Can you work these out from the model? Positions are in its coordinate system, mm. A direction names the side the tool comes from. Give positions to 0.01 mm unless a question says otherwise; leave off trailing zeros. Loops run counter-clockwise (first coordinate to the right, second up) from the corner with the lowest first, then second, coordinate; pieces in that order, holes last. Notation, with made-up numbers: (-12.5, 4.5) - (-2.5, 4.5) arc R19 cw to (-2.5, 31.5) - close; hole circle Ø2 at (32.25, 28). An arc over 180 degrees is marked (long way). Answer as a JSON object with one key per item and string values. Group by question number.
Item 1: Which directions (+Z, -Z, +X, -X, +Y, -Y) give clear straight access to the entire face, cutting with the end or side of a thin tool? Please do faces 1 (the flat face through (24.124, -8, 3)), 2 (the flat face through (13, 25.341, 3)), 3 (the flat face through (91.377, 57, 3)).
Item 2: Thinking about a two-plate mould opening in Y: for faces 4 (the flat face through (90.772, -8, 3)), 5 (the flat face through (48.223, 98.615, 2.958)), 6 (the flat face through (32.043, 67, 3)), which applies, pulls with the +Y half, pulls with the -Y half, needs draft (parallel to the pull), parting line crosses it, or undercut?
Item 3: Suppose I cut it at C-C on z = 2.9. Count the separate pieces of the cut face and the enclosed holes in it, and give its area (3 significant figures).
Item 4: Suppose I cut it at D-D on y = 30. Write out the boundary of the cut face in (x, z).
Item 5: Please list where these lines run through material, in increasing order: L1, parallel to Y at x = 10, z = 3.25; L2, parallel to Y at x = 34.5, z = 3.95; L3, parallel to Y at x = 56.5, z = 5.1.
Item 6: Will these pins go through, and if not, where does the flat tip stop? pin 1 (1.8 mm diameter, centred on y = -7.5, z = 3.5, fed in from +X); pin 2 (2.5 mm diameter, centred on x = 10, z = 4.5, fed in from -Y); pin 3 (1.5 mm diameter, centred on x = 82, z = 2.5, fed in from +Y).
Item 7: Suppose I cut it at B-B on y = 67.5. Write out the boundary of the cut face in (x, z).
Item 8: Suppose I cut it at A-A on x = 14.5. Write out the boundary of the cut face in (y, z).
from build123d import *

# Parameters (mm, degrees)
SKETCH1_W           = 12.2
SKETCH1_H           = 23
BOSS_EXTRUDE1_DEPTH = 6


with BuildPart() as part:
    # Sketch1 → Boss-Extrude1 (new body)
    with BuildSketch(Plane.XY):
        with BuildLine():
            Line((21.077436259, 96.487236066), (24.514288944, 100.118770675))
            ThreePointArc((24.514288944, 100.118770675), (26.133905044, 101.250028723), (28.068821983, 101.648773655))
            Line((28.068821983, 101.648773655), (30.683177697, 101.648773655))
            Line((30.683177697, 101.648773655), (30.683177697, 96.648773655))
            Line((30.683177697, 96.648773655), (33.683177697, 96.648773655))
            Line((33.683177697, 96.648773655), (33.683177697, 101.648773655))
            Line((33.683177697, 101.648773655), (43.068821983, 101.648773655))
            ThreePointArc((43.068821983, 101.648773655), (44.879241743, 101.301597143), (46.432801053, 100.309324643))
            Line((46.432801053, 100.309324643), (50.064335662, 96.872471958))
            ThreePointArc((50.064335662, 96.872471958), (51.617894972, 95.880199458), (53.428314733, 95.533022946))
            Line((53.428314733, 95.533022946), (55.683177697, 95.533022946))
            Line((55.683177697, 95.533022946), (55.683177697, 90.533022946))
            Line((55.683177697, 90.533022946), (58.683177697, 90.533022946))
            Line((58.683177697, 90.533022946), (58.683177697, 95.533022946))
            Line((58.683177697, 95.533022946), (61.489325132, 95.533022946))
            ThreePointArc((61.489325132, 95.533022946), (62.461477954, 95.280855573), (63.188485552, 94.587941837))
            Line((63.188485552, 94.587941837), (66.784051646, 88.796554795))
            ThreePointArc((66.784051646, 88.796554795), (67.511059245, 88.10364106), (68.483212066, 87.851473686))
            Line((68.483212066, 87.851473686), (80.727367549, 87.851473686))
            Line((80.727367549, 87.851473686), (80.727367549, 82.851473686))
            Line((80.727367549, 82.851473686), (83.727367549, 82.851473686))
            Line((83.727367549, 82.851473686), (83.727367549, 87.851473686))
            Line((83.727367549, 87.851473686), (93.887367549, 87.851473686))
            ThreePointArc((93.887367549, 87.851473686), (97.660193959, 86.132598628), (98.839013483, 82.157786039))
            Line((98.839013483, 82.157786039), (90.771737035, 1.27912723))
            Line((90.771737035, 1.27912723), (90.771737035, -16.699114739))
            Line((90.771737035, -16.699114739), (80.611737035, -16.699114739))
            Line((80.611737035, -16.699114739), (80.611737035, 1.27912723))
            Line((80.611737035, 1.27912723), (75.531737035, 1.27912723))
            Line((75.531737035, 1.27912723), (75.531737035, -16.699114739))
            Line((75.531737035, -16.699114739), (67.911737035, -16.699114739))
            Line((67.911737035, -16.699114739), (67.911737035, 1.27912723))
            Line((67.911737035, 1.27912723), (62.831737035, 1.27912723))
            Line((62.831737035, 1.27912723), (62.831737035, -16.699114739))
            Line((62.831737035, -16.699114739), (24.124020717, -16.699114739))
            Line((24.124020717, -16.699114739), (24.124020717, 1.27912723))
            Line((24.124020717, 1.27912723), (19.044020717, 1.27912723))
            Line((19.044020717, 1.27912723), (19.044020717, -16.699114739))
            Line((19.044020717, -16.699114739), (11.424020717, -16.699114739))
            Line((11.424020717, -16.699114739), (11.424020717, 1.27912723))
            Line((11.424020717, 1.27912723), (6.344020717, 1.27912723))
            Line((6.344020717, 1.27912723), (6.344020717, -16.699114739))
            Line((6.344020717, -16.699114739), (-3.815979283, -16.699114739))
            Line((-3.815979283, -16.699114739), (-3.815979283, 1.27912723))
            Line((-3.815979283, 1.27912723), (-3.815979283, 10.864597722))
            Line((-3.815979283, 10.864597722), (8.569519397, 16.399351506))
            Line((8.569519397, 16.399351506), (8.569519397, 20.261157087))
            Line((8.569519397, 20.261157087), (17.062273891, 20.261157087))
            Line((17.062273891, 20.261157087), (17.062273891, 25.341157087))
            Line((17.062273891, 25.341157087), (8.569519397, 25.341157087))
            Line((8.569519397, 25.341157087), (8.569519397, 32.909351506))
            Line((8.569519397, 32.909351506), (17.062273891, 32.909351506))
            Line((17.062273891, 32.909351506), (17.062273891, 37.989351506))
            Line((17.062273891, 37.989351506), (8.569519397, 37.989351506))
            Line((8.569519397, 37.989351506), (8.569519397, 41.799351506))
            Line((8.569519397, 41.799351506), (-3.815979283, 49.840454802))
            Line((-3.815979283, 49.840454802), (-7.075944103, 93.020454802))
            ThreePointArc((-7.075944103, 93.020454802), (-5.26079125, 95.528652506), (-2.316822303, 96.487236066))
            Line((-2.316822303, 96.487236066), (5.683177697, 96.487236066))
            Line((5.683177697, 96.487236066), (5.683177697, 91.487236066))
            Line((5.683177697, 91.487236066), (8.683177697, 91.487236066))
            Line((8.683177697, 91.487236066), (8.683177697, 96.487236066))
            Line((8.683177697, 96.487236066), (21.077436259, 96.487236066))
        make_face()
        with Locations((85.276683747, 57.465671264)):
            Rectangle(SKETCH1_W, SKETCH1_H, mode=Mode.SUBTRACT)
        with Locations((62.066293543, 63.009787098)):
            Rectangle(SKETCH1_W, SKETCH1_H, mode=Mode.SUBTRACT)
        with Locations((38.142588603, 67.50121976)):
            Rectangle(SKETCH1_W, SKETCH1_H, mode=Mode.SUBTRACT)
        with Locations((12.98270306, 64.099542403)):
            Rectangle(SKETCH1_W, SKETCH1_H, mode=Mode.SUBTRACT)
    extrude(amount=BOSS_EXTRUDE1_DEPTH)


solid = part.part
Worked out:
{
 "1": {"face 1": "+Z, -Z, -Y", "face 2": "+Z, -Z, -X", "face 3": "+Z, -Z"},
 "2": {"face 4": "needs draft", "face 5": "pulls with the +Y half", "face 6": "undercut"},
 "3": {"separate pieces": "1", "enclosed holes": "4", "area": "9,010 mm2"},
 "4": {"outline": "(8.57, 0) - (93.64, 0) - (93.64, 6) - (8.57, 6) - close"},
 "5": {"L1": "y = 1.28 to 20.26, 25.34 to 32.91, 37.99 to 52.6, 75.6 to 96.49", "L2": "y = -16.7 to 56, 79 to 101.65", "L3": "y = -16.7 to 51.51, 74.51 to 90.53"},
 "6": {"pin 1": "stops at x = 90.77", "pin 2": "stops at y = 1.28", "pin 3": "stops at y = 82.85"},
 "7": {"outline": "(-5.15, 0) - (6.88, 0) - (6.88, 6) - (-5.15, 6) - close; (19.08, 0) - (32.04, 0) - (32.04, 6) - (19.08, 6) - close; (44.24, 0) - (55.97, 0) - (55.97, 6) - (44.24, 6) - close; (68.17, 0) - (79.18, 0) - (79.18, 6) - (68.17, 6) - close; (91.38, 0) - (97.38, 0) - (97.38, 6) - (91.38, 6) - close"},
 "8": {"outline": "(-16.7, 0) - (20.26, 0) - (20.26, 6) - (-16.7, 6) - close; (25.34, 0) - (32.91, 0) - (32.91, 6) - (25.34, 6) - close; (37.99, 0) - (52.6, 0) - (52.6, 6) - (37.99, 6) - close; (75.6, 0) - (96.49, 0) - (96.49, 6) - (75.6, 6) - close"}
}
